Part model, mm, in its own coordinate system. A direction names the side the tool comes from. Round coordinates to 2 decimals unless told otherwise and drop trailing zeros. Write each loop counter-clockwise with the first axis right and the second up, starting at its lowest first coordinate (ties: lowest second). Pieces come first, ordered by that corner, then holes.
from build123d import *

# Parameters (mm, degrees)
BOSS_EXTRUDE1_DEPTH = 254


with BuildPart() as part:
    # Sketch2 → Boss-Extrude1 (new body)
    with BuildSketch(Plane(origin=(0, 0, 0), x_dir=(1, 0, 0), z_dir=(0, 1, 0))):
        Polygon((-19.05, 19.05), (-4.064, 19.05), (-4.064, 14.986), (-12.112318041, 14.986), (-3.882718041, 6.7564), (3.882718041, 6.7564), (12.112318041, 14.986), (4.064, 14.986), (4.064, 19.05), (19.05, 19.05), (19.05, 4.064), (14.986, 4.064), (14.986, 12.112318041), (6.7564, 3.882718041), (6.7564, -3.882718041), (14.986, -12.112318041), (14.986, -4.064), (19.05, -4.064), (19.05, -19.05), (4.064, -19.05), (4.064, -14.986), (12.112318041, -14.986), (3.882718041, -6.7564), (-3.882718041, -6.7564), (-12.112318041, -14.986), (-4.064, -14.986), (-4.064, -19.05), (-19.05, -19.05), (-19.05, -4.064), (-14.986, -4.064), (-14.986, -12.112318041), (-6.7564, -3.882718041), (-6.7564, 3.882718041), (-14.986, 12.112318041), (-14.986, 4.064), (-19.05, 4.064), align=None)
    extrude(amount=-BOSS_EXTRUDE1_DEPTH)


solid = part.part
Q1. Drop flat-ended pins along their axis: P1, Ø2.5, axis at x = 2, y = -134.5, coming from the +Z side; P2, Ø1, axis at y = -215.5, z = 1, coming from the +X side; P3, Ø6, axis at y = -174.5, z = 0, coming from the -X side. Give the stop position or say it passes through.
Q2. Tool access for faces 5 (the flat face through (17, -125, -4.064)), 6 (the flat face through (0, 0, 0)), 7 (the flat face through (-4.064, -125, 17)): list every direction of +Z, -Z, +X, -X, +Y, -Y with a clear straight run to the whole face (end or side of a thin tool).
Q3. Wall check: line 1 (Z direction, x = 6, y = -20); line 2 (Z direction, x = -15.5, y = -86.5); line 3 (Z direction, x = -11, y = -118). Give the ranges that are in metal, low to high.
Q4. Saw through at B-B, the plane z = 1.5. Write the cut outline in (x, y), and give its area (3 significant figures).
Q5. Saw through at A-A, the plane x = -9. Write the cut outline in (y, z), and give its area (3 significant figures).
Q6. Two-plate mould, pull along Z, no slides. Class faces 1 (the flat face through (-14.986, -125, -8)), 2 (the flat face through (6.756, -125, 0)), 3 (the flat face through (0, -125, -6.756)), 4 (the flat face through (-4.064, -125, -17)): released by +Z, released by -Z, zero draft, split by the parting line, or undercut.
Computed:
1. P1: stops at z = 6.76
1. P2: stops at x = 6.76
1. P3: stops at x = -6.76
2. face 5: +X, +Y, -Y
2. face 6: +Z, -Z, +X, -X, +Y
2. face 7: +Z, +Y, -Y
3. line 1: z = -19.05 to -14.99, -8.87 to 8.87, 14.99 to 19.05
3. line 2: z = -19.05 to -4.06, 4.06 to 19.05
3. line 3: z = -19.05 to -14.99, -13.87 to -8.13, 8.13 to 13.87, 14.99 to 19.05
4. outline: (-6.76, -254) - (6.76, -254) - (6.76, 0) - (-6.76, 0) - close
4. area: 3,430 mm2
5. outline: (-254, -19.05) - (0, -19.05) - (0, -14.99) - (-254, -14.99) - close; (-254, -11.87) - (0, -11.87) - (0, -6.13) - (-254, -6.13) - close; (-254, 6.13) - (0, 6.13) - (0, 11.87) - (-254, 11.87) - close; (-254, 14.99) - (0, 14.99) - (0, 19.05) - (-254, 19.05) - close
5. area: 4,980 mm2
6. face 1: undercut
6. face 2: undercut
6. face 3: released by -Z
6. face 4: zero draft
